```python
from build123d import *

# Parameters (mm, degrees)
SKETCH1_W            = 87.5
SKETCH1_H            = 90
SKETCH1_W_2          = 71.5
SKETCH1_H_2          = 71.5
BOSS_EXTRUDE1_DEPTH  = 5
M4_CLEARANCE_HOLE1_D = 4.5
BOSS_EXTRUDE2_DEPTH  = 90
BOSS_EXTRUDE3_DEPTH  = 87.5
CUT_EXTRUDE1_START   = -81.5
CUT_EXTRUDE1_DEPTH   = 81.5
CUT_EXTRUDE2_START   = -82.75
CUT_EXTRUDE2_DEPTH   = 75.5
SKETCH8_R            = 5
CUT_EXTRUDE3_DEPTH   = 10


with BuildPart() as part:
    # Sketch1 → Boss-Extrude1 (new body)
    with BuildSketch(Plane(origin=(0, 0, 0), x_dir=(0, 0, -1), z_dir=(1, 0, 0))):
        Rectangle(SKETCH1_W, SKETCH1_H)
        Rectangle(SKETCH1_W_2, SKETCH1_H_2, mode=Mode.SUBTRACT)
    extrude(amount=BOSS_EXTRUDE1_DEPTH)

    # M4 Clearance Hole1 (through all)
    with Locations(Plane(origin=(5, 0, 0), x_dir=(0, 0, -1), z_dir=(1, 0, 0))):
        with Locations((-34.25, 42.5), (39.75, 40)):
            m4_clearance_hole1 = Hole(M4_CLEARANCE_HOLE1_D / 2)

    # Mirror1: M4 Clearance Hole1 across plane
    add(m4_clearance_hole1.mirror(Plane.ZX), mode=Mode.SUBTRACT)

    # Sketch4 → Boss-Extrude2 (add)
    with BuildSketch(Plane(origin=(0, 45, 0), x_dir=(1, 0, 0), z_dir=(0, 1, 0))):
        Polygon((5, 35.75), (15, 41.75), (15, 43.75), (5, 37.75), align=None)
        Polygon((5, -35.75), (15, -15.75), (15, -17.75), (5, -37.75), align=None)
    extrude(amount=-BOSS_EXTRUDE2_DEPTH)

    # Sketch5 → Boss-Extrude3 (add)
    with BuildSketch(Plane(origin=(0, 0, -43.75), x_dir=(-1, 0, 0), z_dir=(0, 0, -1))):
        Polygon((-5, 35.75), (-15, 23), (-15, 25), (-5, 37.75), align=None)
        Polygon((-5, -37.75), (-15, -25), (-15, -23), (-5, -35.75), align=None)
    extrude(amount=-BOSS_EXTRUDE3_DEPTH)

    # Sketch6 → Cut-Extrude1 (cut)
    with BuildSketch(Plane(origin=(0, 0, -43.75), x_dir=(-1, 0, 0), z_dir=(0, 0, -1)).offset(CUT_EXTRUDE1_START)):
        Polygon((-5, 45), (-15, 45), (-15, 25), (-5, 37.75), align=None)
        Polygon((-15, -25), (-15, -45), (-5, -45), (-5, -37.75), align=None)
    extrude(amount=CUT_EXTRUDE1_DEPTH, mode=Mode.SUBTRACT)

    # Sketch7 → Cut-Extrude2 (cut)
    with BuildSketch(Plane(origin=(0, 45, 0), x_dir=(1, 0, 0), z_dir=(0, 1, 0)).offset(CUT_EXTRUDE2_START)):
        Polygon((5, -43.75), (15, -43.75), (15, -17.75), (5, -37.75), align=None)
        Polygon((5, 43.75), (15, 43.75), (5, 37.75), align=None)
    extrude(amount=CUT_EXTRUDE2_DEPTH, mode=Mode.SUBTRACT)

    # Sketch8 → Cut-Extrude3 (cut)
    with BuildSketch(Plane(origin=(5, 0, 0), x_dir=(0, 0, -1), z_dir=(1, 0, 0))):
        with Locations((39.75, 40)):
            Circle(SKETCH8_R)
        with Locations((39.75, -40)):
            Circle(SKETCH8_R)
    extrude(amount=CUT_EXTRUDE3_DEPTH, mode=Mode.SUBTRACT)


solid = part.part
```
Build history of the part. All positions in model axes, mm. A direction names the side the tool comes from. Round coordinates to 2 decimals unless told otherwise and drop trailing zeros. Write each loop counter-clockwise with the first axis right and the second up, starting at its lowest first coordinate (ties: lowest second). Pieces come first, ordered by that corner, then holes. Notation, with made-up numbers: (80.5, 60) - (92.5, 60) arc R9 cw to (92.5, 69) - close; hole circle Ø7 at (1, 63.5). An arc over 180 degrees is marked (long way). Write each question's results on one line, items separated by ' | '. Start each with the question number.
Item 1: Mould opens along Z. For faces 5 (the face through (10.07, -0.5, -40.79)), 6 (the face through (2, -1, -35.75)), 7 (the face through (10.07, 0.53, 27.61)), 8 (the face through (2, -35.75, 1)) say: pulls with the +Z half, pulls with the -Z half, needs draft (parallel to the pull), parting line crosses it, or undercut.
Item 2: Saw through at A-A (z = -4). Write the cut outline in (x, y), and give its area (4 significant figures).
Item 3: Drop flat-ended pins along their axis: P1, Ø5, axis at x = 13.5, z = -12, coming from the -Y side; P2, Ø3.5, axis at y = 40, z = -39.75, coming from the -X side; P3, Ø6, axis at x = 10, y = -24.5, coming from the +Z side; P4, Ø1, axis at x = 10.5, y = 1.5, coming from the -Z side. Give the stop position or say it passes through.
Item 4: Saw through at B-B (y = -5). Write the cut outline in (x, z), and give its area (3 significant figures).
Item 5: Saw through at C-C (x = 3). Write the cut outline in (y, z).
Item 6: Wall check: L1, parallel to Y at x = 3.35, z = 34.25; L2, parallel to Y at x = 3.2, z = -39.75; L3, parallel to Z at x = 3, y = -1.5. Give the ranges that are in metal, low to high. Write a range as [from, to].
Item 7: Saw through at D-D (z = 34.25). Write the cut outline in (x, y), and give its area (3 significant figures).
Item 8: Which spindle directions (+Z, -Z, +X, -X, +Y, -Y) get a long thin tool onto all of the face, cutting with end or side? Do faces 1 (the face through (5, 1, 40)), 2 (the face through (2.46, -44.73, 33.96)), 3 (the face through (5.8, 35.7, -37.2)), 4 (the face through (2, -1, 35.75)). Say none if no direction does.
Results are:
1) face 5: pulls with the -Z half | face 6: undercut | face 7: pulls with the +Z half | face 8: undercut
2) outline: (0, -45) - (5, -45) - (5, -37.75) - (15, -25) - (15, -23) - (5, -35.75) - (0, -35.75) - close; (0, 35.75) - (5, 35.75) - (15, 23) - (15, 25) - (5, 37.75) - (5, 45) - (0, 45) - close | area: 132.5 mm²
3) P1: stops at y = -30.1 | P2: passes through | P3: stops at z = 33.75 | P4: stops at z = -41.35
4) outline: (0, -43.75) - (5, -43.75) - (5, -37.75) - (15, -43.75) - (15, -41.75) - (5, -35.75) - (0, -35.75) - close; (0, 35.75) - (5, 35.75) - (15, 15.75) - (15, 17.75) - (5, 37.75) - (5, 43.75) - (0, 43.75) - close | area: 120 mm²
5) outline: (-45, -43.75) - (45, -43.75) - (45, 43.75) - (-45, 43.75) - close; hole circle Ø4.5 at (-42.5, 34.25); hole circle Ø4.5 at (-40, -39.75); hole (-35.75, -35.75) - (35.75, -35.75) - (35.75, 35.75) - (-35.75, 35.75) - close; hole circle Ø4.5 at (40, -39.75); hole circle Ø4.5 at (42.5, 34.25)
6) L1: y = [-45, -44.75], [-40.25, -35.75], [35.75, 40.25], [44.75, 45] | L2: y = [-45, -42.25], [-37.75, 37.75], [42.25, 45] | L3: z = [-43.75, -35.75], [35.75, 43.75]
7) outline: (0, -45) - (5, -45) - (5, -44.75) - (0, -44.75) - close; (0, -40.25) - (5, -40.25) - (5, -37.75) - (6.75, -35.52) - (6.75, 35.52) - (5, 37.75) - (5, 40.25) - (0, 40.25) - (0, 35.75) - (5, 35.75) - (5.75, 34.79) - (5.75, -34.79) - (5, -35.75) - (0, -35.75) - close; (0, 44.75) - (5, 44.75) - (5, 45) - (0, 45) - close | area: 123 mm²
8) face 1: none | face 2: +X, -X | face 3: -Z, +X, +Y | face 4: -X
